Autodesk Inventor part; units mm, degrees
ref_plane "YZ Plane" through (0, 0, 0) normal (1, 0, 0) x (0, 1, 0)
ref_plane "XZ Plane" through (0, 0, 0) normal (0, 1, 0) x (-1, 0, 0)
ref_plane "XY Plane" through (0, 0, 0) normal (0, 0, 1) x (1, 0, 0)
sketch "Sketch1" plane through (0, 0, 0) normal (0, 0, 1) x (1, 0, 0)
  circle A0 centre (0, 0) radius 25.4
  dimension "d0" = 50.8
extrude "Extrusion1" add sketch "Sketch1" along normal blind 304.8
fillet "Fillet1" radius 24.13 1 edges at (-25.4, 0, 304.8)
fillet "Fillet2" radius 24.13 1 edges at (-25.4, 0, 0)
properties part number "Air Tank"
Check sheet for the modelled part. Datum: model origin and axes. Units: mm. Round coordinates to 2 decimals unless told otherwise and drop trailing zeros. Order: outer loops, then holes, each group sorted by start corner. A loop starts at its lowest first (then second) coordinate and runs counter-clockwise, first axis right, second up. Notation, with made-up numbers: M 53,-30.5 L 74,-30.5 A35 ccw 74,2.5 Z; hole C 52.25,41 d2. An arc over 180 degrees is marked long. One line per item, written item: value. Start each with the question number.
1. Gauge pin test, flat ends, axial feed: P1, Ø12, axis at x = 15, z = 248.5, coming from the -Y side; P2, Ø12, axis at y = -8, z = 273, coming from the +X side; P3, Ø5, axis at y = 7.5, z = 169, coming from the -X side. Record the tip position at first contact, or that the pin passes through.
2. Section check A-A on z = 111.5. Enter the section's corners in (x, y).
3. Scan lines: line 1 along X through (y, z) = (-1, 92); line 2 along Y through (x, z) = (1.5, 75.5); line 3 along X through (y, z) = (17, 24). Record each from-to range of solid material in increasing order.
Results found:
1. P1: y = -23.75
1. P2: x = 25.32
1. P3: x = -24.9
2. outline: C 0,0 d50.8
3. line 1: -25.38 to 25.38
3. line 2: -25.36 to 25.36
3. line 3: -18.87 to 18.87
